The listing builds one solid part. Answer for the finished solid, in the listing's coordinates (mm). A direction names the side the tool comes from. Round coordinates to 2 decimals unless told otherwise and drop trailing zeros. Loops run counter-clockwise (first coordinate to the right, second up) from the corner with the lowest first, then second, coordinate; pieces in that order, holes last. Notation, with made-up numbers: M 26,77 L 42,77 A16 cw 42,108 Z; hole C 53.5,-36 d3. An arc over 180 degrees is marked long. Put each result on its own line as item: value. Start each with the question number.
(1) Straight lines are drawn through the part: line 1 (X direction, y = 7.5, z = 32); line 2 (Y direction, x = 18, z = 44); line 3 (Y direction, x = -70, z = 37). For each, find the intervals that lie inside material, in ascending order.
(2) Determine the mould class of faces 4 (the face through (-7.4, 5.86, 34.37)), 5 (the face through (-1, -28.5, 21)), 6 (the face through (-1, 13, 43)) for opening direction Y: released by +Y, released by -Y, zero draft, split by the parting line, or undercut.
(3) Which of the six approach directions +Z, -Z, +X, -X, +Y, -Y give full straight-line access (tool end or side, diameter ignored) to faces 1 (the face through (36.6, 5.86, 34.37)), 2 (the face through (-1, 28.5, 21)), 3 (the face through (86.5, 0, 36))?
(4) Section A-A, the plane z = 32 is taken. Determine the outline of the cut face in (x, y), then the cut area to 3 significant figures.
(5) Section B-B, the plane x = -70 is taken. Determine the outline of the cut face in (y, z).
(6) Flat-ended cylindrical pins translate along their axes: P1, Ø0.9, axis at y = 3, z = 44.5, coming from the -X side; P2, Ø10, axis at x = -31, y = -12.5, coming from the +Z side; P3, Ø2.5, axis at x = 73, z = 45, coming from the +Y side. Find the tip coordinate at first contact, or state that the pin passes through.
```python
from build123d import *

# Parameters (mm, degrees)
SKETCH_W      = 190
SKETCH_H      = 57
PAD_DEPTH     = 43
SKETCH001_R   = 19.5
SKETCH001_W   = 41
SKETCH001_H   = 41
POCKET_DEPTH  = 17.5
SKETCH002_R   = 21.5
SKETCH002_R_2 = 19.268398
SKETCH002_W   = 44.5
SKETCH002_H   = 44.5
SKETCH002_W_2 = 41
SKETCH002_H_2 = 41
PAD001_DEPTH  = 4
FILLET_R      = 1
FILLET001_R   = 3


with BuildPart() as part:
    # Sketch → Pad (new body)
    with BuildSketch(Plane.XY):
        Rectangle(SKETCH_W, SKETCH_H)
    extrude(amount=PAD_DEPTH)

    # Sketch001 (on Face6 of Pad) → Pocket (cut)
    with BuildSketch(Plane.XY.offset(43)):
        with Locations((-70, 0)):
            Circle(SKETCH001_R)
        with Locations((-26, 0)):
            Circle(SKETCH001_R)
        with Locations((18, 0)):
            Circle(SKETCH001_R)
        with Locations((66, 0)):
            Rectangle(SKETCH001_W, SKETCH001_H)
    extrude(amount=-POCKET_DEPTH, mode=Mode.SUBTRACT)

    # Sketch002 (on Face5 of Pocket) → Pad001 (join)
    with BuildSketch(Plane.XY.offset(43)):
        with Locations((-70, 0)):
            Circle(SKETCH002_R)
        with Locations((-70, 0)):
            Circle(SKETCH002_R_2, mode=Mode.SUBTRACT)
        with Locations((-26, 0)):
            Circle(SKETCH002_R)
        with Locations((-26, 0)):
            Circle(SKETCH002_R_2, mode=Mode.SUBTRACT)
        with Locations((18, 0)):
            Circle(SKETCH002_R)
        with Locations((18, 0)):
            Circle(SKETCH002_R_2, mode=Mode.SUBTRACT)
        with Locations((65.887117, 0.207737)):
            Rectangle(SKETCH002_W, SKETCH002_H)
        with Locations((66, 0)):
            Rectangle(SKETCH002_W_2, SKETCH002_H_2, mode=Mode.SUBTRACT)
    extrude(amount=PAD001_DEPTH)

    # Fillet
    fillet_edges = [part.edges().sort_by_distance(p)[0] for p in [
        (-91.5, 0, 47),
        (-47.5, 0, 47),
        (-3.5, 0, 47),
        (65.887117, -22.042263, 47),
        (88.137117, 0.207737, 47),
        (65.887117, 22.457737, 47),
        (43.637117, 0.207737, 47),
    ]]
    fillet(fillet_edges, radius=FILLET_R)

    # Fillet001
    fillet001_edges = [part.edges().sort_by_distance(p)[0] for p in [
        (45.5, -20.5, 34.25),
        (45.5, -20.5, 45),
        (45.5, 20.5, 34.25),
        (45.5, 20.5, 45),
        (86.5, 20.5, 34.25),
        (86.5, -20.5, 34.25),
        (86.5, -20.5, 45),
        (86.5, 20.5, 45),
    ]]
    fillet(fillet001_edges, radius=FILLET001_R)


solid = part.part
```
Recorded:
1. line 1: x = -95 to -88, -52 to -44, -8 to 0, 36 to 45.5, 86.5 to 95
1. line 2: y = -21.5 to -19.27, 19.27 to 21.5
1. line 3: y = -28.5 to -19.5, 19.5 to 28.5
2. face 4: undercut
2. face 5: released by -Y
2. face 6: zero draft
3. face 1: none
3. face 2: +Z, -Z, +X, -X, +Y
3. face 3: +Z
4. outline: M -95,-28.5 L 95,-28.5 L 95,28.5 L -95,28.5 Z; hole C -70,0 d39; hole C -26,0 d39; hole C 18,0 d39; hole M 45.5,-17.5 A3 ccw 48.5,-20.5 L 83.5,-20.5 A3 ccw 86.5,-17.5 L 86.5,17.5 A3 ccw 83.5,20.5 L 48.5,20.5 A3 ccw 45.5,17.5 Z
4. area: 5,570 mm²
5. outline: M -28.5,0 L 28.5,0 L 28.5,43 L 21.5,43 L 21.5,46 A1 ccw 20.5,47 L 19.27,47 L 19.27,43 L 19.5,43 L 19.5,25.5 L -19.5,25.5 L -19.5,43 L -19.27,43 L -19.27,47 L -20.5,47 A1 ccw -21.5,46 L -21.5,43 L -28.5,43 Z
6. P1: stops at x = -91.35
6. P2: stops at z = 25.5
6. P3: stops at y = 22.46
